Autodesk Inventor part; units mm, degrees
ref_plane "YZ Plane" through (0, 0, 0) normal (1, 0, 0) x (0, 1, 0)
ref_plane "XZ Plane" through (0, 0, 0) normal (0, 1, 0) x (-1, 0, 0)
ref_plane "XY Plane" through (0, 0, 0) normal (0, 0, 1) x (1, 0, 0)
sketch "Sketch1" plane through (0, 0, 0) normal (0, 1, 0) x (-1, 0, 0)
  line L0 (0, 0) -> (38.1, 0)
  line L1 (38.1, 0) -> (38.1, -241.3)
  line L2 (38.1, -241.3) -> (0, -241.3)
  line L3 (0, -241.3) -> (0, 0)
  dimension "d0" = 38.1
  dimension "d1" = 241.3
extrude "Extrusion1" add sketch "Sketch1" along normal blind 19.05
sketch "Sketch2" plane through (0, 0, -241.3) normal (0, 0, -1) x (-1, 0, 0)
  line L0 (204.3257, -100.8201) -> (38.1, 11.3005)
  line L1 (38.1, 11.3005) -> (31.5757, 0)
  line L2 (0, 0) -> (38.1, 0)
  line L3 (38.1, 11.3005) -> (51.1487, 11.3005) construction
  line L4 (31.5757, 0) -> (38.1, 0)
  line L5 (38.1, 0) -> (38.1, 11.3005)
  dimension "d4" = 120
extrude "Extrusion2" cut sketch "Sketch2" against normal blind 241.3
properties part number "front_screen_footer"
Work out the finished part from the listing and answer in its coordinate system (mm). Give positions to 0.01 mm unless a question says otherwise; leave off trailing zeros. Write each loop counter-clockwise with the first axis right and the second up, starting at its lowest first coordinate (ties: lowest second). Pieces come first, ordered by that corner, then holes. Notation, with made-up numbers: (72.5, -31.5) - (128.5, -31.5) arc R6 cw to (128.5, -24.5) - close; hole circle Ø9 at (-17, 62.25). An arc over 180 degrees is marked (long way). One line per item, written item: value. Start each with the question number.
1. Given pin 1 (10 mm diameter, centred on x = -11, y = 12.5, fed in from +Z), flat-ended and moving along its own axis, determine where the tip first touches the part or whether it passes through.
2. Find section A-A (z = -146). Write down the section's boundary in (x, y), then the cut area to 3 significant figures.
3. Find section B-B (y = 9). Write down the section's boundary in (x, z), then the cut area to 3 significant figures.
4. Consider probe 1 along X at (y, z) = (3.25, -110.5); probe 2 along X at (y, z) = (10.75, -205.5); probe 3 along Y at (x, z) = (-33, -219.5). Determine where each line is inside the solid, lowest interval first.
Geometry results:
1. pin 1: z = 0
2. outline: (-38.1, 11.3) - (-31.58, 0) - (0, 0) - (0, 19.05) - (-38.1, 19.05) - close
2. area: 689 mm2
3. outline: (-36.77, -241.3) - (0, -241.3) - (0, 0) - (-36.77, 0) - close
3. area: 8,870 mm2
4. probe 1: -33.45 to 0
4. probe 2: -37.78 to 0
4. probe 3: 2.47 to 19.05
